Autodesk Inventor part; units mm, degrees
ref_plane "Plano de trabalho1" through (0, 0, 4) normal (0, 0, 1) x (1, 0, 0)
ref_plane "YZ Plane" through (0, 0, 0) normal (1, 0, 0) x (0, 1, 0)
ref_plane "XZ Plane" through (0, 0, 0) normal (0, 1, 0) x (-1, 0, 0)
sketch "Esboço1" plane through (0, 0, 0) normal (1, 0, 0) x (0, 1, 0)
  circle A0 centre (0, 0) radius 4
  dimension "d0" = 8
extrude "Extrusão1" add sketch "Esboço1" along normal blind 45
fillet "Arredondamento1" radius 1 1 edges at (45, -4, 0)
ref_plane "Plano de trabalho1" through (0, 0, 4) normal (0, 0, 1) x (1, 0, 0)
sketch "Esboço2" plane through (0, 0, 4) normal (0, 0, 1) x (1, 0, 0)
  line L0 (45, 3) -> (45, -3)
  line L1 (45, 0) -> (40, 0)
  point P0 (0, 0)
  dimension "d5" = 5
hole "Furo1" at (40, 0, 4) direction (0, 0, -1) diameter 3 end through all
properties part number "piston"
For this review, take the finished solid that the model builds, in its own axes (mm). Round coordinates to 2 decimals unless told otherwise and drop trailing zeros. Write each loop counter-clockwise with the first axis right and the second up, starting at its lowest first coordinate (ties: lowest second). Pieces come first, ordered by that corner, then holes. Notation, with made-up numbers: (-5, -27) - (26, -27) arc R8 ccw to (26, -22) - close; hole circle Ø8 at (9, 50.25). An arc over 180 degrees is marked (long way). Put each result on its own line as item: value.
Q1. Insertion check: pin 1 Ø3 at (x, z) = (6.5, 3) entering from +Y; pin 2 Ø1.5 at (x, y) = (7.5, 2.5) entering from -Z; pin 3 Ø4 at (x, y) = (28, -3) entering from +Z. Each pin has a flat end and moves straight along its axis. Give the tip position at first contact, or say it passes through.
Solved:
pin 1: stops at y = 3.71
pin 2: stops at z = -3.6
pin 3: stops at z = 3.87
Q2. We need section D-D (x = 30). Give the boundary of the cut face in (y, z), and give its area (3 significant figures).
Solved:
outline: circle Ø8 at (0, 0)
area: 50.3 mm2
Q3. Wall thickness on probe 1 along X at (y, z) = (0, -2.25); probe 2 along X at (y, z) = (-1.25, 1.75); probe 3 along Z at (x, y) = (12, -0.25): over which ranges is each line inside the solid? List them lowest first.
Solved:
probe 1: x = 0 to 38.5, 41.5 to 45
probe 2: x = 0 to 39.17, 40.83 to 45
probe 3: z = -3.99 to 3.99
Q4. We need section A-A (y = 0). Give the boundary of the cut face in (x, z).
Solved:
outline: (0, -4) - (38.5, -4) - (38.5, 4) - (0, 4) - close; (41.5, -4) - (44, -4) arc R1 ccw to (45, -3) - (45, 3) arc R1 ccw to (44, 4) - (41.5, 4) - close
Q5. We need section B-B (z = 0). Give the boundary of the cut face in (x, y).
Solved:
outline: (0, -4) - (44, -4) arc R1 ccw to (45, -3) - (45, 3) arc R1 ccw to (44, 4) - (0, 4) - close; hole circle Ø3 at (40, 0)
Q6. Mouldability with a two-part tool opening along Y and no side actions: class faces 1 (the face through (21.692, -0.867, 3.905)), 2 (the face through (41.464, 0.325, -0.056)), 3 (the face through (0, 0, 0)) as released by +Y, released by -Y, zero draft, split by the parting line, or undercut.
Solved:
face 1: split by the parting line
face 2: undercut
face 3: zero draft
Q7. We need section C-C (x = 40). Give the boundary of the cut face in (y, z), and give its area (3 significant figures).
Solved:
outline: (-1.5, -3.71) - (-1.5, 3.71) arc R4 ccw to start; (1.5, -3.71) arc R4 ccw to (1.5, 3.71) - close
area: 26.8 mm2
